```python
from build123d import *

# Parameters (mm, degrees)
SKETCH1_R           = 67.8
SKETCH1_R_2         = 50
BOSS_EXTRUDE1_DEPTH = 10
SKETCH2_R           = 25
BOSS_EXTRUDE2_DEPTH = 20
SKETCH3_R           = 67.8
CUT_EXTRUDE1_DEPTH  = 10
SKETCH4_R           = 50
CUT_EXTRUDE2_DEPTH  = 11
SKETCH5_W           = 15.080994576
SKETCH5_H           = 20
CUT_EXTRUDE3_DEPTH  = 21
SKETCH6_W           = 19.646297403
SKETCH6_H           = 20
CUT_EXTRUDE4_DEPTH  = 21


with BuildPart() as part:
    # Sketch1 → Boss-Extrude1 (new body)
    with BuildSketch(Plane.XY):
        Circle(SKETCH1_R)
        Circle(SKETCH1_R_2, mode=Mode.SUBTRACT)
    extrude(amount=BOSS_EXTRUDE1_DEPTH)

    # Sketch2 → Boss-Extrude2 (add)
    with BuildSketch(Plane.XY):
        with BuildLine():
            ThreePointArc((-63.772719488, 46.746532272), (-8.415408503, 77.65917808), (50.844425579, 55.113765796))
            ThreePointArc((50.844425579, 55.113765796), (96.256515498, 24.521091043), (150, 35))
            ThreePointArc((150, 35), (185, 0), (150, -35))
            ThreePointArc((150, -35), (96.256515498, -24.521091043), (50.844425579, -55.113765796))
            ThreePointArc((50.844425579, -55.113765796), (-8.415408503, -77.65917808), (-63.772719488, -46.746532272))
            ThreePointArc((-63.772719488, -46.746532272), (-104.453573255, -23.015011619), (-150, -35))
            ThreePointArc((-150, -35), (-185, 0), (-150, 35))
            ThreePointArc((-150, 35), (-104.453573255, 23.015011619), (-63.772719488, 46.746532272))
        make_face()
        with Locations((-150, 0)):
            Circle(SKETCH2_R, mode=Mode.SUBTRACT)
        with Locations((150, 0)):
            Circle(SKETCH2_R, mode=Mode.SUBTRACT)
    extrude(amount=BOSS_EXTRUDE2_DEPTH)

    # Sketch3 → Cut-Extrude1 (cut)
    with BuildSketch(Plane.XY.offset(20)):
        Circle(SKETCH3_R)
    extrude(amount=-CUT_EXTRUDE1_DEPTH, mode=Mode.SUBTRACT)

    # Sketch4 → Cut-Extrude2 (cut, through all)
    with BuildSketch(Plane.XY.offset(10)):
        Circle(SKETCH4_R)
    extrude(amount=-CUT_EXTRUDE2_DEPTH, mode=Mode.SUBTRACT)

    # Sketch5 → Cut-Extrude3 (cut, through all)
    with BuildSketch(Plane.XY.offset(20)):
        with Locations((-180.419979471, -0.076174623)):
            Rectangle(SKETCH5_W, SKETCH5_H)
    extrude(amount=-CUT_EXTRUDE3_DEPTH, mode=Mode.SUBTRACT)

    # Sketch6 → Cut-Extrude4 (cut, through all)
    with BuildSketch(Plane.XY.offset(20)):
        with Locations((179.499488159, -2.442655022)):
            Rectangle(SKETCH6_W, SKETCH6_H)
    extrude(amount=-CUT_EXTRUDE4_DEPTH, mode=Mode.SUBTRACT)


solid = part.part
```
Work out the finished part from the listing and answer in its coordinate system (mm). A direction names the side the tool comes from. Coordinates: 2 decimals unless noted, no trailing zeros. Loops run counter-clockwise (first coordinate to the right, second up) from the corner with the lowest first, then second, coordinate; pieces in that order, holes last. Notation, with made-up numbers: M 73.25,-7 L 83.25,-7 A5 cw 83.25,0 Z; hole C -28.75,6.25 d8. An arc over 180 degrees is marked long. Use CSV: the item, a comma, the result in double quotes. Start each with the question number.
(1) For faces 1 (the face through (-7.5, -77.72, 9.86)), 2 (the face through (-178, 9.924, 10)), 3 (the face through (-49.971, 45.822, 15.07)), 4 (the face through (177, -12.443, 10)), determine the directions among +Z, -Z, +X, -X, +Y, -Y from which every point of the face is accessible in a straight line to the end or side of a thin tool.
(2) Find section C-C, the plane y = 0. Give the vertices of the cut face in (x, z).
(3) Find section B-B, the plane z = 4.5. Give the vertices of the cut face in (x, y), then the cut area to 3 significant figures.
(4) Consider line 1 (Y direction, x = 0, z = 5.5); line 2 (X direction, y = 16, z = 16); line 3 (Y direction, x = -150, z = 12). Determine where each line is inside the solid, lowest interval first.
(5) Find section D-D, the plane x = -110. Give the vertices of the cut face in (y, z).
(6) Given pin 1 Ø5.5 at (x, z) = (-179, 10) entering from -Y; pin 2 Ø1 at (x, z) = (-101, 6) entering from -Y; pin 3 Ø5.5 at (x, z) = (176.5, 8) entering from +Y, each flat-ended and moving along its own axis, determine where each tip first touches the part or whether it passes through.
(7) For a pull along Y with two mould halves and no side action, classify faces 5 (the face through (-103.78, -23.11, 9.86)), 6 (the face through (42, 29, 0)), 7 (the face through (179, 7.557, 10)) as +Y half, -Y half, draft (parallel to the pull), parting line (faces both ways), or undercut.
(8) Find section A-A, the plane x = 0. Give the vertices of the cut face in (y, z), then the cut area to 3 significant figures.
Recorded:
1,face 1,"+Z, -Z, -Y"
1,face 2,"+Z, -Z, -X"
1,face 3,"+Z"
1,face 4,"+Z, -Z, +X"
2,outline,"M -125,0 L -50,0 L -50,10 L -67.8,10 L -67.8,20 L -125,20 Z; M 50,0 L 125,0 L 125,20 L 67.8,20 L 67.8,10 L 50,10 Z"
3,outline,"M -183.56,9.92 L -172.95,9.92 A25 cw long -172.88,-10.08 L -183.52,-10.08 A35 ccw -150,-35 A61.54 cw -63.77,-46.75 A75 ccw 50.84,-55.11 A71.54 cw 150,-35 A35 ccw 182.71,-12.44 L 171.68,-12.44 A25 cw long 173.83,7.56 L 184.17,7.56 A35 ccw 150,35 A71.54 cw 50.84,55.11 A75 ccw -63.77,46.75 A61.54 cw -150,35 A35 ccw Z; hole C 0,0 d100"
3,area,"18,500 mm^2"
4,line 1,"y = -77.8 to -50, 50 to 77.8"
4,line 2,"x = -181.13 to -169.21, -130.79 to -65.89, 65.89 to 130.79, 169.21 to 181.13"
4,line 3,"y = -35 to -25, 25 to 35"
5,outline,"M -22.51,0 L 22.51,0 L 22.51,20 L -22.51,20 Z"
6,pin 1,"stops at y = -23.15"
6,pin 2,"stops at y = -23.69"
6,pin 3,"stops at y = 25.71"
7,face 5,"-Y half"
7,face 6,"draft"
7,face 7,"undercut"
8,outline,"M -77.8,0 L -50,0 L -50,10 L -67.8,10 L -67.8,20 L -77.8,20 Z; M 50,0 L 77.8,0 L 77.8,20 L 67.8,20 L 67.8,10 L 50,10 Z"
8,area,"756 mm^2"
